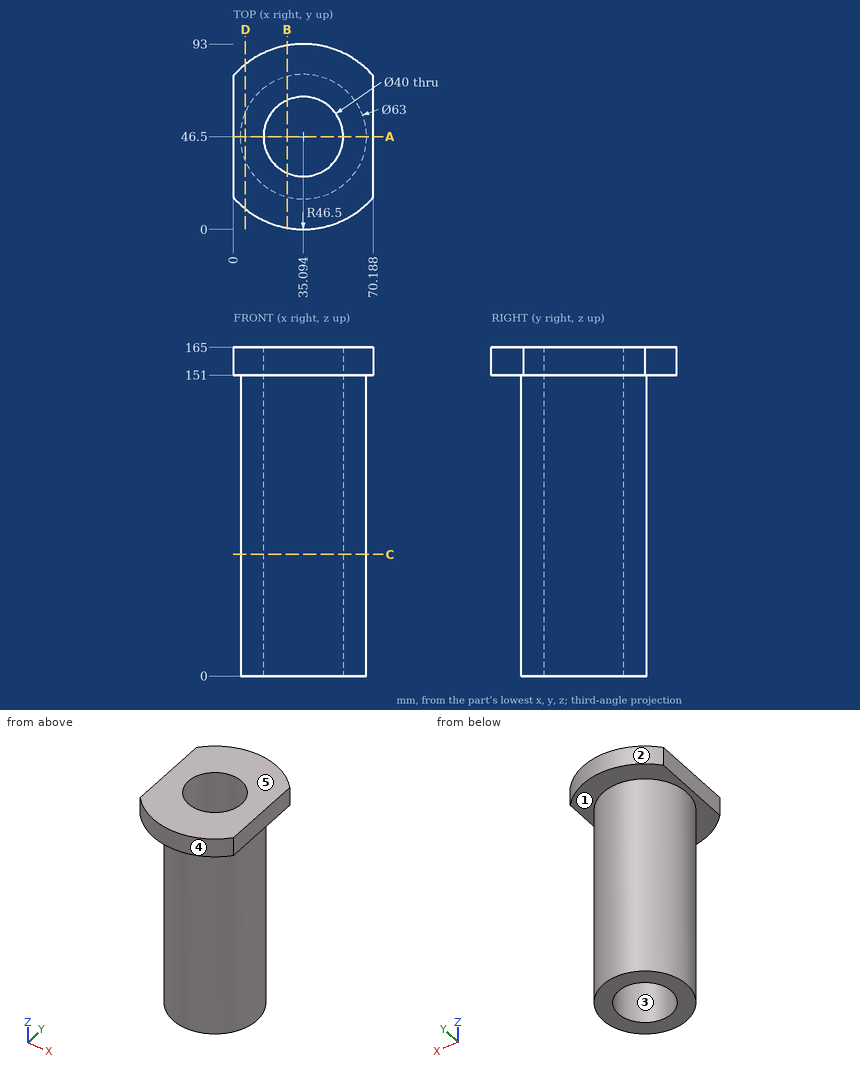
Print and shaded views of the part. All mm, measured from the part's lowest x, y and z. A direction names the side the tool comes from. Give positions to 0.01 mm unless a question says otherwise; leave off trailing zeros. Loops run counter-clockwise (first coordinate to the right, second up) from the corner with the lowest first, then second, coordinate; pieces in that order, holes last. Notation, with made-up numbers: (62.25, -19.5) - (121.25, -19.5) arc R35 ccw to (121.25, 13.5) - close; hole circle Ø9 at (41.5, 81). An arc over 180 degrees is marked (long way). Use a Markdown table: item, result.
(1) Band-saw the part on C-C (z = 61). Give the cut face in (x, y), and give its area (3 significant figures).
Taken from the geometry:
| item | result |
|---|---|
| outline | circle Ø63 at (35.09, 46.5); hole circle Ø40 at (35.09, 46.5) |
| area | 1,860 mm2 |
(2) Drop flat-ended pins along their axis: pin 1 Ø2 at (x, z) = (53.5, 70.5) entering from -Y; pin 2 Ø3 at (y, z) = (42, 129) entering from +X; pin 3 Ø4 at (y, z) = (26, 69.5) entering from -X. Give the stop position or say it passes through.
Taken from the geometry:
| item | result |
|---|---|
| pin 1 | y = 20.25 |
| pin 2 | x = 66.45 |
| pin 3 | x = 9.6 |
(3) Band-saw the part on B-B (x = 27). Give the cut face in (y, z), and give its area (3 significant figures).
Taken from the geometry:
| item | result |
|---|---|
| outline | (0.71, 151) - (16.06, 151) - (16.06, 0) - (28.21, 0) - (28.21, 165) - (0.71, 165) - close; (64.79, 0) - (76.94, 0) - (76.94, 151) - (92.29, 151) - (92.29, 165) - (64.79, 165) - close |
| area | 4,440 mm2 |
(4) Band-saw the part on D-D (x = 6). Give the cut face in (y, z).
Taken from the geometry:
| item | result |
|---|---|
| outline | (10.23, 151) - (34.43, 151) - (34.43, 0) - (58.57, 0) - (58.57, 151) - (82.77, 151) - (82.77, 165) - (10.23, 165) - close |
(5) Pull direction Y, two halves, no side cores. Call the marked faces 3, 4 and 5: +Y half, -Y half, draft (parallel to the pull), parting line (faces both ways), or undercut.
Taken from the geometry:
| item | result |
|---|---|
| face 3 | undercut |
| face 4 | -Y half |
| face 5 | draft |
(6) Which spindle directions (+Z, -Z, +X, -X, +Y, -Y) get a long thin tool onto all of the face, cutting with end or side? Do the marked faces 1 and 2. Say none if no direction does.
Taken from the geometry:
| item | result |
|---|---|
| face 1 | -Z |
| face 2 | +Z, -Z, +Y |
(7) Wall check: line 1 along X through (y, z) = (46, 46); line 2 along Y through (x, z) = (35, 144); line 3 along X through (y, z) = (60.5, 18.5). Give the ranges that are in metal, low to high.
Taken from the geometry:
| item | result |
|---|---|
| line 1 | 3.6 to 15.1, 55.09 to 66.59 |
| line 2 | 15 to 26.5, 66.5 to 78 |
| line 3 | 6.88 to 20.81, 49.38 to 63.31 |
(8) Band-saw the part on A-A (y = 46.5). Give the cut face in (x, z).
Taken from the geometry:
| item | result |
|---|---|
| outline | (0, 151) - (3.59, 151) - (3.59, 0) - (15.09, 0) - (15.09, 165) - (0, 165) - close; (55.09, 0) - (66.59, 0) - (66.59, 151) - (70.19, 151) - (70.19, 165) - (55.09, 165) - close |
